Work out the finished part from the listing and answer in its coordinate system (mm). Face numbers are marked on the shaded views. A direction names the side the tool comes from. Round coordinates to 2 decimals unless told otherwise and drop trailing zeros. Order: outer loops, then holes, each group sorted by start corner. A loop starts at its lowest first (then second) coordinate and runs counter-clockwise, first axis right, second up. Notation, with made-up numbers: (5, -36.5) - (24, -36.5) arc R29 cw to (24, -1.5) - close; hole circle Ø7 at (11.5, 31). An arc over 180 degrees is marked (long way). Answer in a Markdown table with one row per item.
from build123d import *

# Parameters (mm, degrees)
SKETCH1_W           = 25
SKETCH1_H           = 10
BOSS_EXTRUDE1_DEPTH = 15
SKETCH2_W           = 20
SKETCH2_H           = 10
CUT_EXTRUDE1_DEPTH  = 6
SKETCH3_W           = 9
SKETCH3_H           = 10
CUT_EXTRUDE2_DEPTH  = 6.5
SKETCH4_W           = 15.5
SKETCH4_H           = 10
CUT_EXTRUDE3_DEPTH  = 3.5


with BuildPart() as part:
    # Sketch1 → Boss-Extrude1 (new body)
    with BuildSketch(Plane.XY):
        Rectangle(SKETCH1_W, SKETCH1_H)
    extrude(amount=BOSS_EXTRUDE1_DEPTH)

    # Sketch2 → Cut-Extrude1 (cut)
    with BuildSketch(Plane.XY.offset(15)):
        Rectangle(SKETCH2_W, SKETCH2_H)
    extrude(amount=-CUT_EXTRUDE1_DEPTH, mode=Mode.SUBTRACT)

    # Sketch3 → Cut-Extrude2 (cut)
    with BuildSketch(Plane.XY.offset(9)):
        Rectangle(SKETCH3_W, SKETCH3_H)
    extrude(amount=-CUT_EXTRUDE2_DEPTH, mode=Mode.SUBTRACT)

    # Sketch4 → Cut-Extrude3 (cut)
    with BuildSketch(Plane.XY.offset(9)):
        Rectangle(SKETCH4_W, SKETCH4_H)
    extrude(amount=-CUT_EXTRUDE3_DEPTH, mode=Mode.SUBTRACT)


solid = part.part
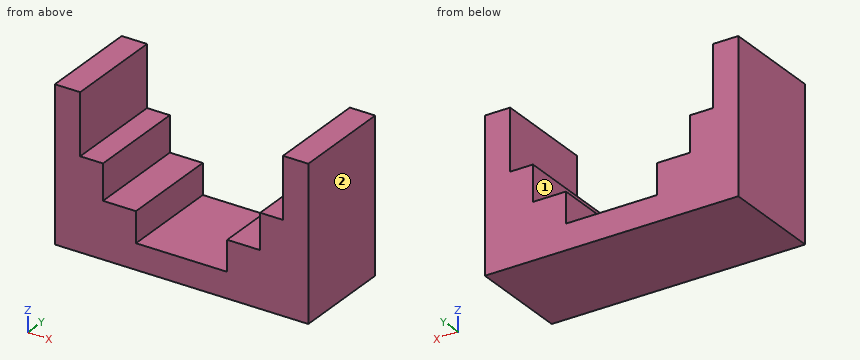
1) Which of the six approach directions +Z, -Z, +X, -X, +Y, -Y give full straight-line access (tool end or side, diameter ignored) to the marked faces 1 and 2?
Filled in:
| item | result |
|---|---|
| face 1 | +Z, +Y, -Y |
| face 2 | +Z, -Z, +X, +Y, -Y |
2) Each of these flat-tipped pins is pushed along its axis until it touches: pin 1 (1 mm diameter, centred on x = 6, y = 2, fed in from +Z); pin 2 (6 mm diameter, centred on x = 5.5, y = 0, fed in from +Z); pin 3 (2.5 mm diameter, centred on x = 1, y = 2.5, fed in from +Z). Where does it stop, or does it pass through?
Filled in:
| item | result |
|---|---|
| pin 1 | stops at z = 5.5 |
| pin 2 | stops at z = 9 |
| pin 3 | stops at z = 2.5 |
3) Find section A-A, the plane z = 10. Give the vertices of the cut face in (x, y).
Filled in:
| item | result |
|---|---|
| outline | (-12.5, -5) - (-10, -5) - (-10, 5) - (-12.5, 5) - close; (10, -5) - (12.5, -5) - (12.5, 5) - (10, 5) - close |
4) Find section C-C, the plane y = -0.75. Give the vertices of the cut face in (x, z).
Filled in:
| item | result |
|---|---|
| outline | (-12.5, 0) - (12.5, 0) - (12.5, 15) - (10, 15) - (10, 9) - (7.75, 9) - (7.75, 5.5) - (4.5, 5.5) - (4.5, 2.5) - (-4.5, 2.5) - (-4.5, 5.5) - (-7.75, 5.5) - (-7.75, 9) - (-10, 9) - (-10, 15) - (-12.5, 15) - close |
5) Find the intervals of material crossed by probe 1 along X at (y, z) = (-1.25, 3.5); probe 2 along X at (y, z) = (-1.5, 6.25); probe 3 along Z at (x, y) = (0, -0.25), in increasing order. Write a range as from..to.
Filled in:
| item | result |
|---|---|
| probe 1 | x = -12.5..-4.5, 4.5..12.5 |
| probe 2 | x = -12.5..-7.75, 7.75..12.5 |
| probe 3 | z = 0..2.5 |
6) Find section B-B, the plane z = 3.25. Give the vertices of the cut face in (x, y), then the cut area to 3 significant figures.
Filled in:
| item | result |
|---|---|
| outline | (-12.5, -5) - (-4.5, -5) - (-4.5, 5) - (-12.5, 5) - close; (4.5, -5) - (12.5, -5) - (12.5, 5) - (4.5, 5) - close |
| area | 160 mm^2 |
7) Find section D-D, the plane x = -1.75. Give the vertices of the cut face in (y, z), then the cut area to 3 significant figures.
Filled in:
| item | result |
|---|---|
| outline | (-5, 0) - (5, 0) - (5, 2.5) - (-5, 2.5) - close |
| area | 25.0 mm^2 |
